from build123d import *

# Parameters (mm, degrees)
BOSS_EXTRUDE1_DEPTH       = 18.25625
F_1_1_69_DIAMETER_HOLE1_D = 42.926


with BuildPart() as part:
    # Sketch1 → Boss-Extrude1 (new body)
    with BuildSketch(Plane(origin=(0, 0, 0), x_dir=(1, 0, 0), z_dir=(0, 1, 0))):
        Polygon((2032, 450.85), (457.2, 990.6), (0, 990.6), (0, 0), (2032, 0), align=None)
    extrude(amount=BOSS_EXTRUDE1_DEPTH)

    # 1 (1.69) Diameter Hole1 (through all)
    with Locations(Plane(origin=(0, 18.25625, 0), x_dir=(1, 0, 0), z_dir=(0, 1, 0))):
        with Locations((1524, 88.9), (914.4, 478.79), (304.8, 868.68)):
            Hole(F_1_1_69_DIAMETER_HOLE1_D / 2)


solid = part.part
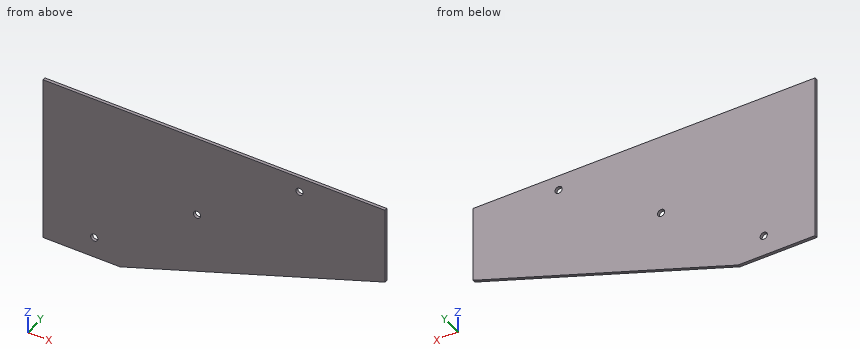
The model under review builds one solid part; all positions refer to its coordinate system, in mm. Give positions to 0.01 mm unless a question says otherwise; leave off trailing zeros. Loops run counter-clockwise (first coordinate to the right, second up) from the corner with the lowest first, then second, coordinate; pieces in that order, holes last. Notation, with made-up numbers: (69, 45.5) -> (107, 45.5) arc R31 ccw to (107, 81.5) -> close; hole circle Ø6 at (36.25, 48). An arc over 180 degrees is marked (long way). Put each result on its own line as item: value. Start each with the question number.
1. Wall thickness on probe 1 along X at (y, z) = (7, -88.9); probe 2 along Z at (x, y) = (914.4, 7.25); probe 3 along Z at (x, y) = (1524, 14): over which ranges is each line inside the solid? List them lowest first.
2. We need section D-D on x = 1296.5. State the section outline as (y, z) points.
3. We need section A-A on z = -88.9. State the section outline as (x, y) points, then the cut area to 3 significant figures.
4. We need section B-B on x = 914.4. State the section outline as (y, z) points.
5. Clearance check with flat-ended pins moving along their axes: P1, Ø5, axis at x = 602, y = 15.5, coming from the +Z side; P2, Ø1.5, axis at x = 1143, y = 14.5, coming from the -Z side; P3, Ø4, axis at x = 983, y = 7, coming from the -Z side. State where each tip first meets the part, or that it passes through.
6. We need section C-C on y = 9.75. State the section outline as (x, z) points, then the cut area to 3 significant figures.
Determined:
1. probe 1: 0 to 1502.54, 1545.46 to 2032
1. probe 2: -833.9 to -500.25, -457.33 to 0
1. probe 3: -624.96 to -110.36, -67.44 to 0
2. outline: (0, -702.94) -> (18.26, -702.94) -> (18.26, 0) -> (0, 0) -> close
3. outline: (0, 0) -> (1502.54, 0) -> (1502.54, 18.26) -> (0, 18.26) -> close; (1545.46, 0) -> (2032, 0) -> (2032, 18.26) -> (1545.46, 18.26) -> close
3. area: 36,300 mm^2
4. outline: (0, -833.9) -> (18.26, -833.9) -> (18.26, -500.25) -> (0, -500.25) -> close; (0, -457.33) -> (18.26, -457.33) -> (18.26, 0) -> (0, 0) -> close
5. P1: z = 0
5. P2: z = -755.8
5. P3: z = -811.07
6. outline: (0, -990.6) -> (457.2, -990.6) -> (2032, -450.85) -> (2032, 0) -> (0, 0) -> close; hole circle Ø42.93 at (304.8, -868.68); hole circle Ø42.93 at (914.4, -478.79); hole circle Ø42.93 at (1524, -88.9)
6. area: 1,580,000 mm^2
